Part model, mm, in its own coordinate system. A direction names the side the tool comes from. Give positions to 0.01 mm unless a question says otherwise; leave off trailing zeros. Write each loop counter-clockwise with the first axis right and the second up, starting at its lowest first coordinate (ties: lowest second). Pieces come first, ordered by that corner, then holes. Notation, with made-up numbers: M 84,-25.5 L 111,-25.5 A13 cw 111,-9.5 Z; hole C -10,73.25 d1. An arc over 180 degrees is marked long. Use CSV: the item, a comma, the result in double quotes. Start each with the question number.
1. Drill centre lines: line 1 along Y through (x, z) = (0, 1.4); line 2 along Y through (x, z) = (0, 2.35); line 3 along Y through (x, z) = (-1.5, 2.3). Where is each one in solid material? Low to high. Write a range as from..to.
2. 3-axis set-ups, long thin cutter, end or side, ignore diameter. For faces 1 (the face through (-0.59, 4.46, 2.51)), 2 (the face through (1.6, -4.9, 3)), 3 (the face through (1.08, -4.88, 0.49)): which of +Z, -Z, +X, -X, +Y, -Y reach the whole face in a straight line?
3. Mould opens along X. For faces 4 (the face through (3.233, -1.341, 1.479)), 5 (the face through (-1.08, -4.88, 2.51)), 6 (the face through (0, -4, 3)), 7 (the face through (-1.19, -5.37, 1.48)) say: pulls with the +X half, pulls with the -X half, needs draft (parallel to the pull), parting line crosses it, or undercut.
4. Band-saw the part on D-D, the plane z = 1.7. List the corners of the cut face in (x, y), then the cut area to 3 significant figures.
5. Drop a flat-ended pin along its axis: pin 1 Ø6.5 at (x, y) = (0, 0) entering from +Z. Give the stop position or say it passes through.
6. Band-saw the part on A-A, the plane x = 0. List the corners of the cut face in (y, z), then the cut area to 3 significant figures.
7. Band-saw the part on C-C, the plane z = 2.35. List the corners of the cut face in (x, y), then the cut area to 3 significant figures.
from build123d import *

# Parameters (mm, degrees)
SKETCH_1_R          = 5.5
SKETCH_1_R_2        = 3.5
EXTRUDE_1_DEPTH     = 3
SKETCH_2_R          = 5
SKETCH_2_R_2        = 4.5
CUT_EXTRUDE_1_DEPTH = 1
SKETCH_3_R          = 5
SKETCH_3_R_2        = 4.5
CUT_EXTRUDE_2_DEPTH = 1


with BuildPart() as part:
    # 草图1 → 凸台-拉伸1 (new body)
    with BuildSketch(Plane.XY):
        Circle(SKETCH_1_R)
        Circle(SKETCH_1_R_2, mode=Mode.SUBTRACT)
    extrude(amount=EXTRUDE_1_DEPTH)

    # 草图2 → 切除-拉伸1 (cut)
    with BuildSketch(Plane.XY.offset(3)):
        Circle(SKETCH_2_R)
        Circle(SKETCH_2_R_2, mode=Mode.SUBTRACT)
    extrude(amount=-CUT_EXTRUDE_1_DEPTH, mode=Mode.SUBTRACT)

    # 草图3 → 切除-拉伸2 (cut)
    with BuildSketch(Plane(origin=(0, 0, 0), x_dir=(-1, 0, 0), z_dir=(0, 0, -1))):
        Circle(SKETCH_3_R)
        Circle(SKETCH_3_R_2, mode=Mode.SUBTRACT)
    extrude(amount=-CUT_EXTRUDE_2_DEPTH, mode=Mode.SUBTRACT)


solid = part.part
Output:
1,line 1,"y = -5.5..-3.5, 3.5..5.5"
1,line 2,"y = -5.5..-5, -4.5..-3.5, 3.5..4.5, 5..5.5"
1,line 3,"y = -5.29..-4.77, -4.24..-3.16, 3.16..4.24, 4.77..5.29"
2,face 1,"+Z"
2,face 2,"+Z, +X, -X, +Y, -Y"
2,face 3,"-Z"
3,face 4,"undercut"
3,face 5,"undercut"
3,face 6,"needs draft"
3,face 7,"parting line crosses it"
4,outline,"C 0,0 d11; hole C 0,0 d7"
4,area,"56.5 mm²"
5,pin 1,"passes through"
6,outline,"M -5.5,0 L -5,0 L -5,1 L -4.5,1 L -4.5,0 L -3.5,0 L -3.5,3 L -4.5,3 L -4.5,2 L -5,2 L -5,3 L -5.5,3 Z; M 3.5,0 L 4.5,0 L 4.5,1 L 5,1 L 5,0 L 5.5,0 L 5.5,3 L 5,3 L 5,2 L 4.5,2 L 4.5,3 L 3.5,3 Z"
6,area,"10.0 mm²"
7,outline,"C 0,0 d11; C 0,0 d9; hole C 0,0 d10; hole C 0,0 d7"
7,area,"41.6 mm²"
